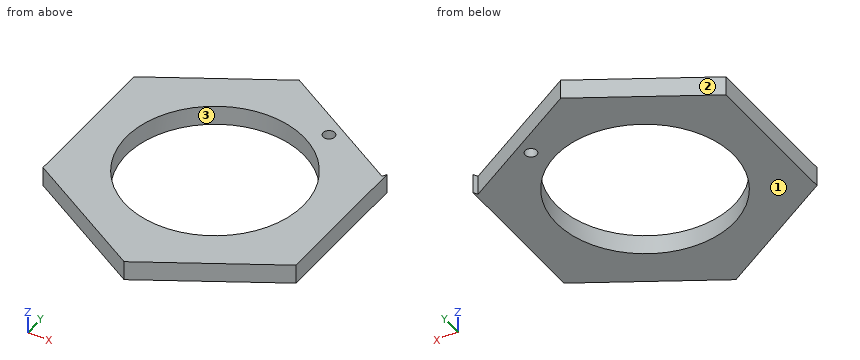
from build123d import *

# Parameters (mm, degrees)
SKETCH_R   = 9.1
SKETCH_R_2 = 0.6
PAD_DEPTH  = 2


with BuildPart() as part:
    # Sketch → Pad (new body)
    with BuildSketch(Plane.XY):
        Polygon((-0.50397, 14.713397), (-12.984903, 7.508821), (-12.99, -7.5), (0, -14.99967), (12.99, -7.5), (12.99, 7.5), (12.74, 7.066987), align=None)
        Circle(SKETCH_R, mode=Mode.SUBTRACT)
        with Locations((5.747722, 9.571406)):
            Circle(SKETCH_R_2, mode=Mode.SUBTRACT)
    extrude(amount=PAD_DEPTH)


solid = part.part
Can you work these out from the model? Positions are in its coordinate system, mm. Face numbers are marked on the shaded views. Round coordinates to 2 decimals unless told otherwise and drop trailing zeros. Write each loop counter-clockwise with the first axis right and the second up, starting at its lowest first coordinate (ties: lowest second). Pieces come first, ordered by that corner, then holes. Notation, with made-up numbers: (-26.5, 78.25) -> (-3.5, 78.25) arc R29 cw to (-3.5, 103.25) -> close; hole circle Ø6 at (66.25, 9.25). An arc over 180 degrees is marked (long way). Use one line per item in the form item = value. Start each with the question number.
Q1. I'm going to push a flat-ended pin straight in: P1, Ø1, axis at x = 3, z = 1, coming from the -Y side. Where does the tip first touch, or does it pass through?
Q2. Imagine slicing it at A-A (x = -1). Please give me the cut outline in (y, z).
Q3. We'd pull the mould along Y, two halves only. Please class the marked faces 1, 2 and 3: +Y half, -Y half, draft (parallel to the pull), parting line (faces both ways), or undercut.
Q4. Imagine slicing it at B-B (y = 6.75). Please give me the cut outline in (x, z).
Q5. Imagine slicing it at D-D (y = 10.75). Please give me the cut outline in (x, z).
Q6. Imagine slicing it at C-C (z = 0.55). Please give me the cut outline in (x, y), then the cut area to 3 significant figures.
Q7. If I drill on probe 1 along Y at (x, z) = (5.5, 1.65); probe 2 along Y at (x, z) = (-6.25, 0.7); probe 3 along Y at (x, z) = (0.75, 0.15), over which ranges is the centre line in solid material (lowest first)? Write a range as [from, to].
Worked out:
q1.P1 = -13.56
q2.outline = (-14.42, 0) -> (-9.04, 0) -> (-9.04, 2) -> (-14.42, 2) -> close; (9.04, 0) -> (14.43, 0) -> (14.43, 2) -> (9.04, 2) -> close
q3.face_1 = draft
q3.face_2 = +Y half
q3.face_3 = undercut
q4.outline = (-12.99, 0) -> (-6.1, 0) -> (-6.1, 2) -> (-12.99, 2) -> close; (6.1, 0) -> (12.99, 0) -> (12.99, 2) -> (6.1, 2) -> close
q5.outline = (-7.37, 0) -> (6.36, 0) -> (6.36, 2) -> (-7.37, 2) -> close
q6.outline = (-12.99, -7.5) -> (0, -15) -> (12.99, -7.5) -> (12.99, 7.5) -> (12.74, 7.07) -> (-0.5, 14.71) -> (-12.98, 7.51) -> close; hole circle Ø18.2 at (0, 0); hole circle Ø1.2 at (5.75, 9.57)
q6.area = 316 mm^2
q7.probe_1 = [-11.82, -7.25], [7.25, 9.02], [10.12, 11.25]
q7.probe_2 = [-11.39, -6.61], [6.61, 11.4]
q7.probe_3 = [-14.57, -9.07], [9.07, 13.99]
